Input: part model. Units: mm. Frame: model coordinates. Face numbers are marked on the shaded views. A direction names the side the tool comes from. Round coordinates to 2 decimals unless told otherwise and drop trailing zeros. Order: outer loops, then holes, each group sorted by start corner. A loop starts at its lowest first (then second) coordinate and runs counter-clockwise, first axis right, second up.
Item 1: Line query: L1, parallel to X at y = 0, z = -2.3; L2, parallel to Y at x = 0, z = 0; L3, parallel to X at y = -3, z = 25.5. Output: solid intervals per line, ascending.
Item 2: First-contact query: pin 1 (6 mm diameter, centred on y = -35, z = 17, fed in from +X); pin 2 (3 mm diameter, centred on x = 19.5, z = 4.5, fed in from -Y); pin 3 (3.5 mm diameter, centred on x = -22.5, y = -1, fed in from -Z); pin 4 (4.5 mm diameter, centred on x = 0.5, y = -30, fed in from -Z). Flat tips, straight axial feed; report the tip coordinate or a pass-through.
Item 3: Mould query, pull axis Z, two halves, no side actions, for the marked faces 6, 7 and 8. Classes: released by +Z, released by -Z, zero draft, split by the parting line, or undercut.
Item 4: Cut plane A-A on z = 8.5. Give the number of separate pieces and of enclosed holes in the cut face, then the cut area to 3 significant figures.
Item 5: Reachability of the marked faces 1, 2, 3, 4 and 5 from +Z, -Z, +X, -X, +Y, -Y: full face, straight path, thin tool, end or side. Return the list, or none.
Item 6: Cut plane D-D on x = 25.5. Output: boundary loops of the cut face in (y, z).
Item 7: Cut plane C-C on y = -11. Output: boundary loops of the cut face in (x, z), then the cut area to 3 significant figures.
```python
from build123d import *

# Parameters (mm, degrees)
F0_W            = 91.5
F0_H            = 7
F1_DEPTH        = 5
F2_W            = 5
F2_H            = 40.75
F3_DEPTH        = 3.5
F4_W            = 4
F4_H            = 10
F5_DEPTH        = 37.5
F6_W            = 4
F6_H            = 10
F7_DEPTH        = 37.5
F8_W            = 10
F8_H            = 7
F9_DEPTH        = 37.5
F10_W           = 10
F10_H           = 4
F11_DEPTH       = 9
F12_W           = 10
F12_H           = 4
F13_DEPTH       = 9
F14_W           = 10
F14_H           = 4
F15_DEPTH       = 9
F16_R           = 1.99999
F18_D           = 2
F18_DEPTH       = 18
F18_CSINK_D     = 4
F18_CSINK_ANGLE = 82
F18_TIP         = 0.600860619
F19_W           = 3
F19_H           = 10
F20_DEPTH       = 3
F21_R           = 1
F22_W           = 5
F22_H           = 27.7060836997
F23_DEPTH       = 0.5


# Not quite as in the source:
# - a fillet or chamfer is up to 0.001 mm smaller than in the source, because OpenCascade refuses the exact size


with BuildPart() as f1:
    # F0 (on Front) → F1 (new body, symmetric)
    with BuildSketch(Plane.XZ):
        Rectangle(F0_W, F0_H)
    extrude(amount=F1_DEPTH, both=True)

    # F2 (on Top) → F3 (join, symmetric)
    with BuildSketch(Plane.XY):
        with Locations((-2.5, -20.375)):
            Rectangle(F2_W, F2_H)
        with Locations((2.5, -20.375)):
            Rectangle(F2_W, F2_H)
    extrude(amount=F3_DEPTH, both=True)

    # F4 (on face) → F5 (join)
    with BuildSketch(Plane.XY.offset(3.5)):
        with Locations((-43.75, 0)):
            Rectangle(F4_W, F4_H)
    extrude(amount=F5_DEPTH)

    # F6 (on face) → F7 (join)
    with BuildSketch(Plane.XY.offset(3.5)):
        with Locations((43.75, 0)):
            Rectangle(F6_W, F6_H)
    extrude(amount=F7_DEPTH)

    # F8 (on face) → F9 (join)
    with BuildSketch(Plane.XY.offset(3.5)):
        with Locations((0, -37.25)):
            Rectangle(F8_W, F8_H)
    extrude(amount=F9_DEPTH)

    # F10 (on face) → F11 (join)
    with BuildSketch(Plane(origin=(0, -33.75, 0), x_dir=(-1, 0, 0), z_dir=(0, 1, 0))):
        with Locations((0, 39)):
            Rectangle(F10_W, F10_H)
    extrude(amount=F11_DEPTH)

    # F12 (on face) → F13 (join)
    with BuildSketch(Plane(origin=(41.75, 0, 0), x_dir=(0, -1, 0), z_dir=(-1, 0, 0))):
        with Locations((0, 39)):
            Rectangle(F12_W, F12_H)
    extrude(amount=F13_DEPTH)

    # F14 (on face) → F15 (join)
    with BuildSketch(Plane.YZ.offset(-41.75)):
        with Locations((0, 39)):
            Rectangle(F14_W, F14_H)
    extrude(amount=F15_DEPTH)

    # F16 (radius 2 in the source; OpenCascade refuses exactly that, so slightly less here)
    f16_edges = [f1.edges().sort_by_distance(p)[0] for p in [
        (0, 5, 3.5),
        (41.75, 5, 20.25),
        (37.25, 5, 37),
        (-41.75, 5, 20.25),
        (-37.25, 5, 37),
        (32.75, 0, 41),
        (39.25, 5, 41),
        (45.75, 5, 18.75),
        (-45.75, 5, 18.75),
        (-39.25, 5, 41),
        (-32.75, 0, 41),
        (0, -24.75, 41),
        (-5, -33.75, 20.25),
        (5, -33.75, 20.25),
        (-41.75, -5, 20.25),
        (41.75, -5, 20.25),
        (-37.25, -5, 37),
        (37.25, -5, 37),
        (-45.75, 0, 41),
        (45.75, 0, 41),
        (0, -40.75, 41),
        (5, -32.75, 41),
        (-5, -32.75, 41),
        (0, -24.75, 37),
        (-5, -40.75, 18.75),
        (5, -40.75, 18.75),
        (39.25, -5, 41),
        (-39.25, -5, 41),
        (-45.75, -5, 18.75),
        (45.75, -5, 18.75),
        (-32.75, 0, 37),
        (32.75, 0, 37),
    ]]
    fillet(f16_edges, radius=F16_R)

    # F18
    with Locations(Plane.XY.offset(3.5)):
        with Locations((0, 0)):
            CounterSinkHole(F18_D / 2, F18_CSINK_D / 2, depth=F18_DEPTH, counter_sink_angle=F18_CSINK_ANGLE)
            with Locations((0, 0, -(F18_DEPTH + F18_TIP / 2))):  # 118° drill point
                Cone(0, F18_D / 2, F18_TIP, mode=Mode.SUBTRACT)

    # F19 (on face) → F20 (cut)
    with BuildSketch(Plane(origin=(0, 0, -3.5), x_dir=(1, 0, 0), z_dir=(0, 0, -1))):
        with Locations((21.5, 0)):
            Rectangle(F19_W, F19_H)
        with Locations((-22.5, 0)):
            Rectangle(F19_W, F19_H)
    extrude(amount=-F20_DEPTH, mode=Mode.SUBTRACT)

    # F21
    f21_edges = [f1.edges().sort_by_distance(p)[0] for p in [
        (20, 0, -3.5),
        (23, 0, -3.5),
        (-21, 0, -3.5),
        (-24, 0, -3.5),
    ]]
    fillet(f21_edges, radius=F21_R)

    # F22 (on face) → F23 (cut)
    with BuildSketch(Plane(origin=(0, 0, -3.5), x_dir=(1, 0, 0), z_dir=(0, 0, -1))):
        with Locations((0, 18.8530418498)):
            Rectangle(F22_W, F22_H)
    extrude(amount=-F23_DEPTH, mode=Mode.SUBTRACT)


solid = f1.part
```
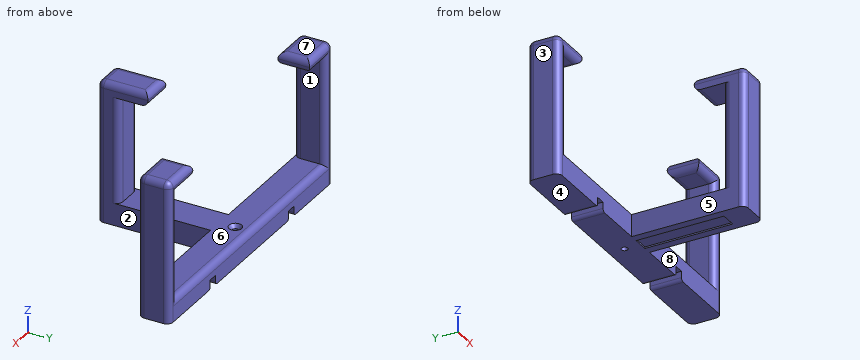
From the geometry:
1. L1: x = -45.75 to -24, -21 to -1, 1 to 20, 23 to 45.75
1. L2: y = -40.75 to -1, 1 to 5
1. L3: x = -45.75 to -41.75, 41.75 to 45.75
2. pin 1: stops at x = 5
2. pin 2: stops at y = -5
2. pin 3: stops at z = -3.16
2. pin 4: stops at z = -3.5
3. face 6: undercut
3. face 7: released by +Z
3. face 8: zero draft
4. separate pieces: 3
4. enclosed holes: 0
4. area: 140 mm2
5. face 1: +Y, -Y
5. face 2: +Z, -Z, +X, -Y
5. face 3: +Z, -Z, -X, +Y, -Y
5. face 4: -Z, +X, -X, +Y, -Y
5. face 5: +Z, -Z, -X, -Y
6. outline: (-5, -3.5) - (5, -3.5) - (5, 1.5) arc R2 ccw to (3, 3.5) - (-5, 3.5) - close
7. outline: (-5, -3.5) - (-2.5, -3.5) - (-2.5, -3) - (2.5, -3) - (2.5, -3.5) - (5, -3.5) - (5, 3.5) - (-5, 3.5) - close
7. area: 67.5 mm2
